```python
from build123d import *

# Parameters (mm, degrees)
SKETCH1_W           = 304.8
SKETCH1_H           = 100
SKETCH1_R           = 4.05
BOSS_EXTRUDE1_DEPTH = 6.35


with BuildPart() as part:
    # Sketch1 → Boss-Extrude1 (new body)
    with BuildSketch(Plane(origin=(0, 0, 0), x_dir=(1, 0, 0), z_dir=(0, 1, 0))):
        with Locations((152.4, 50)):
            Rectangle(SKETCH1_W, SKETCH1_H)
        with Locations(Location((40, 65, 0), (0, 0, 270))):
            Circle(SKETCH1_R, mode=Mode.SUBTRACT)
        with Locations(Location((120, 65, 0), (0, 0, 270))):
            Circle(SKETCH1_R, mode=Mode.SUBTRACT)
        with Locations(Location((200, 65, 0), (0, 0, 270))):
            Circle(SKETCH1_R, mode=Mode.SUBTRACT)
        with Locations(Location((280, 65, 0), (0, 0, 270))):
            Circle(SKETCH1_R, mode=Mode.SUBTRACT)
    extrude(amount=-BOSS_EXTRUDE1_DEPTH)


solid = part.part
```
Geometry: final body of the model. Coordinates: model frame, mm. Give positions to 0.01 mm unless a question says otherwise; leave off trailing zeros. Order: outer loops, then holes, each group sorted by start corner. A loop starts at its lowest first (then second) coordinate and runs counter-clockwise, first axis right, second up. Notation, with made-up numbers: (-1, -7) -> (56, -7) arc R20 ccw to (56, 20) -> close; hole circle Ø10 at (66.25, 21). An arc over 180 degrees is marked (long way). Write each question's results on one line, items separated by ' | '. Start each with the question number.
1) Draft query along X for faces 1 (the flat face through (304.8, -3, -49)), 2 (the cylindrical face through (276.407, -3.131, -63.131)), 3 (the flat face through (150, -6.35, -51)), 4 (the flat face through (0, -3, -49)). Return one class per face: pulls with the +X half, pulls with the -X half, needs draft (parallel to the pull), parting line crosses it, or undercut.
2) Section A-A (x = 40). Return loops of the section in (y, z).
3) Section B-B (z = -65). Return loops of the section in (x, y), then the cut area to 3 significant figures.
4) Line query: line 1 (X direction, y = -3, z = -65); line 2 (Z direction, x = 280, y = -2); line 3 (Z direction, x = 196.5, y = -2.25). Output: solid intervals per line, ascending. Write a range as from..to.
5) First-contact query: pin 1 (6.5 mm diameter, centred on x = 280, z = -65, fed in from +Y). Flat tip, straight axial feed; report the tip coordinate or a pass-through.
Calculated:
1) face 1: pulls with the +X half | face 2: undercut | face 3: needs draft | face 4: pulls with the -X half
2) outline: (-6.35, -100) -> (0, -100) -> (0, -69.05) -> (-6.35, -69.05) -> close; (-6.35, -60.95) -> (0, -60.95) -> (0, 0) -> (-6.35, 0) -> close
3) outline: (0, -6.35) -> (35.95, -6.35) -> (35.95, 0) -> (0, 0) -> close; (44.05, -6.35) -> (115.95, -6.35) -> (115.95, 0) -> (44.05, 0) -> close; (124.05, -6.35) -> (195.95, -6.35) -> (195.95, 0) -> (124.05, 0) -> close; (204.05, -6.35) -> (275.95, -6.35) -> (275.95, 0) -> (204.05, 0) -> close; (284.05, -6.35) -> (304.8, -6.35) -> (304.8, 0) -> (284.05, 0) -> close | area: 1,730 mm2
4) line 1: 0..35.95, 44.05..115.95, 124.05..195.95, 204.05..275.95, 284.05..304.8 | line 2: -100..-69.05, -60.95..0 | line 3: -100..-67.04, -62.96..0
5) pin 1: through
